Could you check a few things on this drawing? It's one solid part, dimensions in mm from its lowest x, y, z. Round coordinates to 2 decimals unless told otherwise and drop trailing zeros. Loops run counter-clockwise (first coordinate to the right, second up) from the corner with the lowest first, then second, coordinate; pieces in that order, holes last. Notation, with made-up numbers: M 3.25,1 L 61.25,1 A27 ccw 61.25,26 Z; hole C 87,75 d5. An arc over 180 degrees is marked long. Answer as CSV lines item,"result".
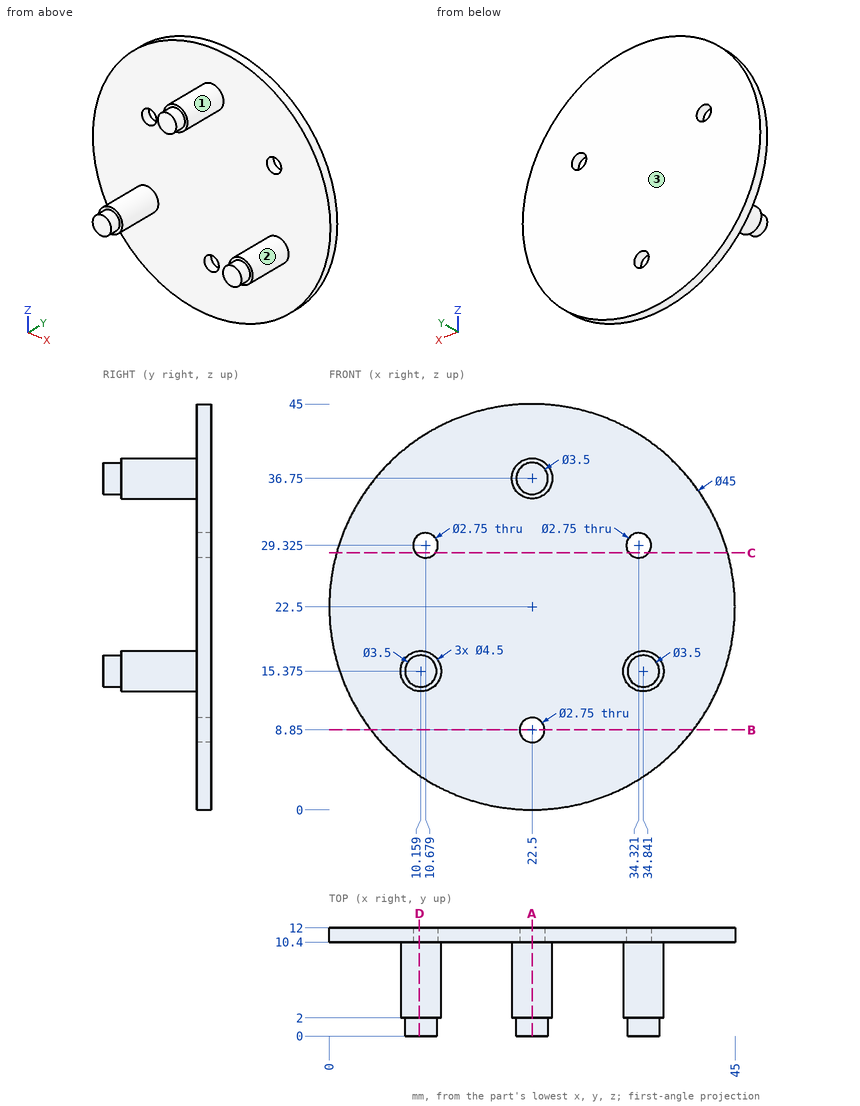
Item 1: We'd pull the mould along X, two halves only. Please class the marked faces 1, 2 and 3: released by +X, released by -X, zero draft, split by the parting line, or undercut.
Output:
face 1,"split by the parting line"
face 2,"undercut"
face 3,"zero draft"
Item 2: If we section it at B-B on z = 8.85: Write out the boundary of the cut face in (x, y) (1 decimal).
Output:
outline,"M 4.6,10.4 L 21.1,10.4 L 21.1,12 L 4.6,12 Z; M 23.9,10.4 L 40.4,10.4 L 40.4,12 L 23.9,12 Z"
Item 3: If we section it at D-D on x = 10: Write out the boundary of the cut face in (y, z).
Output:
outline,"M 0,13.63 L 2,13.63 L 2,13.13 L 10.4,13.13 L 10.4,3.79 L 12,3.79 L 12,28.13 L 10.4,28.13 L 10.4,17.62 L 2,17.62 L 2,17.12 L 0,17.12 Z; M 10.4,30.52 L 12,30.52 L 12,41.21 L 10.4,41.21 Z"
Item 4: If we section it at C-C on z = 28.5: Write out the boundary of the cut face in (x, y) (1 decimal).
Output:
outline,"M 0.8,10.4 L 9.6,10.4 L 9.6,12 L 0.8,12 Z; M 11.8,10.4 L 33.2,10.4 L 33.2,12 L 11.8,12 Z; M 35.4,10.4 L 44.2,10.4 L 44.2,12 L 35.4,12 Z"
Item 5: Will these pins go through, and if not, where does the flat tip stop? pin 1 (3 mm diameter, centred on x = 37.5, z = 5.5, fed in from -Y); pin 2 (5 mm diameter, centred on x = 25.5, y = 7.5, fed in from +Z); pin 3 (1.5 mm diameter, centred on x = 11, y = 10.5, fed in from +Z); pin 4 (6 mm diameter, centred on x = 16, y = 3.5, fed in from +Z).
Output:
pin 1,"stops at y = 10.4"
pin 2,"stops at z = 38.94"
pin 3,"stops at z = 42.27"
pin 4,"passes through"
Item 6: If I drill on line 1 along Z through (x, y) = (22.5, 11.3) (1 decimal); line 2 along Y through (x, z) = (29, 30); line 3 along Y through (x, z) = (8, 15), over which ranges is the centre line in solid material (lowest first)? Write a range as from..to.
Output:
line 1,"z = 0..7.5, 10.2..45"
line 2,"y = 10.4..12"
line 3,"y = 2..12"
Item 7: If we section it at A-A on x = 22.5: Write out the boundary of the cut face in (y, z) (1 decimal), then the cut area to 3 significant figures.
Output:
outline,"M 0,35 L 2,35 L 2,34.5 L 10.4,34.5 L 10.4,10.2 L 12,10.2 L 12,45 L 10.4,45 L 10.4,39 L 2,39 L 2,38.5 L 0,38.5 Z; M 10.4,0 L 12,0 L 12,7.5 L 10.4,7.5 Z"
area,"112 mm2"
